The model under review builds one solid part; all positions refer to its coordinate system, in mm. Face numbers are marked on the shaded views. A direction names the side the tool comes from. Give positions to 0.01 mm unless a question says otherwise; leave off trailing zeros. Order: outer loops, then holes, each group sorted by start corner. A loop starts at its lowest first (then second) coordinate and runs counter-clockwise, first axis right, second up. Notation, with made-up numbers: (19, 22.25) - (43, 22.25) arc R14 cw to (43, 26.25) - close; hole circle Ø1 at (63.5, 46.5). An arc over 180 degrees is marked (long way). Use a Markdown table: item, result. Add a question column.
```python
from build123d import *

# Parameters (mm, degrees)
SKETCH2_R          = 1.5
CUT_EXTRUDE1_DEPTH = 10.2


with BuildPart() as part:
    # Sketch1 → Revolve1 (revolve)
    with BuildSketch(Plane.XY):
        Polygon((13, 0), (13, -3), (5, -3), (5, -9.2), (3, -9.2), (3, -6.2), (0, -6.2), (0, 0), align=None)
    revolve(axis=Axis((0, 0, 0), (0, 1, 0)))

    # Sketch2 → Cut-Extrude1 (cut, through all)
    with BuildSketch(Plane(origin=(0, 0, 0), x_dir=(1, 0, 0), z_dir=(0, 1, 0))):
        with Locations((9, 0)):
            Circle(SKETCH2_R)
        with Locations((-9, 0)):
            Circle(SKETCH2_R)
    extrude(amount=-CUT_EXTRUDE1_DEPTH, mode=Mode.SUBTRACT)


solid = part.part
```
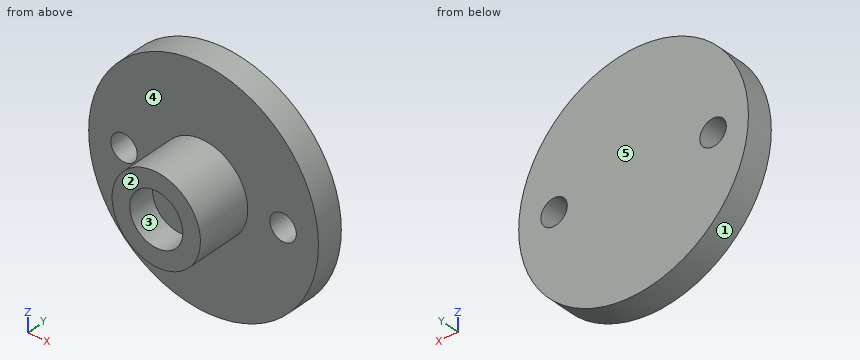
Q1. We need section D-D (y = -5). Write out the cut boundary in (x, z), plus the area to 3 significant figures.
Q2. Wall thickness on probe 1 along X at (y, z) = (-2.2, 0); probe 2 along Z at (x, y) = (0, -7.65); probe 3 along Y at (x, z) = (8, 1.25): over which ranges is each line inside the solid? List them lowest first.
Q3. We need section B-B (x = 0). Write out the cut boundary in (y, z), plus the area to 3 significant figures.
Q4. We need section A-A (z = 0). Write out the cut boundary in (x, y).
Q5. Clearance check with flat-ended pins moving along their axes: P1, Ø3, axis at x = 0, z = 1, coming from the -Y side; P2, Ø4, axis at x = -9, z = 0, coming from the -Y side; P3, Ø1.5, axis at y = -5, z = -6, coming from the -X side; P4, Ø1, axis at x = 2.5, y = -3, coming from the -Z side. State where each tip first meets the part, or that it passes through.
Q6. Machinability: for the marked faces 4 and 5, which of the approach directions +Z, -Z, +X, -X, +Y, -Y give a long, thin tool a straight path to every point of the face, cutting with its end or side? Answer none if there is none.
Q7. Draft analysis for pull direction X (two halves, no side actions). For the marked faces 1, 2 and 3, state which applies: pulls with the +X half, pulls with the -X half, needs draft (parallel to the pull), parting line crosses it, or undercut.
Q8. We need section C-C (x = 9). Write out the cut boundary in (y, z), plus the area to 3 significant figures.
Here are the results:
| question | item | result |
|---|---|---|
| 1 | outline | circle Ø10 at (0, 0) |
| 1 | area | 78.5 mm2 |
| 2 | probe 1 | -13 to -10.5, -7.5 to 7.5, 10.5 to 13 |
| 2 | probe 2 | -5 to -3, 3 to 5 |
| 2 | probe 3 | -3 to 0 |
| 3 | outline | (-9.2, -5) - (-3, -5) - (-3, -13) - (0, -13) - (0, 13) - (-3, 13) - (-3, 5) - (-9.2, 5) - (-9.2, 3) - (-6.2, 3) - (-6.2, -3) - (-9.2, -3) - close |
| 3 | area | 122 mm2 |
| 4 | outline | (-13, -3) - (-10.5, -3) - (-10.5, 0) - (-13, 0) - close; (-7.5, -3) - (-5, -3) - (-5, -9.2) - (-3, -9.2) - (-3, -6.2) - (3, -6.2) - (3, -9.2) - (5, -9.2) - (5, -3) - (7.5, -3) - (7.5, 0) - (-7.5, 0) - close; (10.5, -3) - (13, -3) - (13, 0) - (10.5, 0) - close |
| 5 | P1 | y = -6.2 |
| 5 | P2 | y = -3 |
| 5 | P3 | through |
| 5 | P4 | z = -12.85 |
| 6 | face 4 | -Y |
| 6 | face 5 | +Z, -Z, +X, -X, +Y |
| 7 | face 1 | parting line crosses it |
| 7 | face 2 | needs draft |
| 7 | face 3 | undercut |
| 8 | outline | (-3, -9.38) - (0, -9.38) - (0, -1.5) - (-3, -1.5) - close; (-3, 1.5) - (0, 1.5) - (0, 9.38) - (-3, 9.38) - close |
| 8 | area | 47.3 mm2 |
